```python
from build123d import *

# Parameters (mm, degrees)
F1_DEPTH      = 25.4
F1_DEPTH_BACK = 25.4
F3_D          = 5.1054


with BuildPart() as f1:
    # F0 (on Front) → F1 (new body, two sides)
    with BuildSketch(Plane.XZ) as f1_sk:
        Polygon((733.425, 292.1), (-733.425, 292.1), (-733.425, -292.1), (-682.625, -292.1), (-682.625, 241.3), (682.625, 241.3), (682.625, -292.1), (733.425, -292.1), align=None)
    extrude(amount=F1_DEPTH)
    extrude(f1_sk.sketch, amount=-F1_DEPTH_BACK)

    # F3 (through all)
    with Locations(Plane.XZ.offset(25.4)):
        with Locations((-708.025, -50.8), (708.025, -50.8), (708.025, 69.85), (-708.025, 69.85)):
            Hole(F3_D / 2)


solid = f1.part
```
Can you work these out from the model? Positions are in its coordinate system, mm. A direction names the side the tool comes from. Coordinates: 2 decimals unless noted, no trailing zeros. Order: outer loops, then holes, each group sorted by start corner. A loop starts at its lowest first (then second) coordinate and runs counter-clockwise, first axis right, second up.
1. Thinking about a two-plate mould opening in X: for faces 3 (the face through (-10, 0, 241.3)), 4 (the face through (-708, 0, -292.1)), 5 (the face through (-733.425, 0, 4)), 6 (the face through (733.425, 0, -4)), which applies, +X half, -X half, draft (parallel to the pull), parting line (faces both ways), or undercut?
2. If we section it at A-A (z = -70.5): Please give me the cut outline in (x, y) (3 decimals), then the cut area to 3 significant figures.
3. If we section it at C-C (x = 276): Please give me the cut outline in (y, z), then the cut area to 3 significant figures.
4. I need wall thicknesses on line 1 (X direction, y = 0, z = 69) (3 decimals); line 2 (X direction, y = 18, z = 122) (3 decimals); line 3 (Z direction, x = -478, y = 13.5). Which ranges of each line are inside material? Lowest first, please.
5. If we section it at B-B (y = -4): Please give me the cut outline in (x, z) (3 decimals).
6. For faces 1 (the face through (-682.625, 0, -29)), 2 (the face through (708, 0, -292.1)), which set-ups out of +Z, -Z, +X, -X, +Y, -Y let a thin tool reach every point of the face, with its end or its side?
7. I'm going to push flat-ended pins straight in: pin 1 (15 mm diameter, centred on x = -262, y = -9.5, fed in from -Z); pin 2 (4 mm diameter, centred on x = 708.025, z = -50.8, fed in from +Y); pin 3 (6.5 mm diameter, centred on x = -708.025, z = 69.85, fed in from +Y). Where does each tip first touch, or does it pass through?
Entries:
1. face 3: undercut
1. face 4: draft
1. face 5: -X half
1. face 6: +X half
2. outline: (-733.425, -25.4) - (-682.625, -25.4) - (-682.625, 25.4) - (-733.425, 25.4) - close; (682.625, -25.4) - (733.425, -25.4) - (733.425, 25.4) - (682.625, 25.4) - close
2. area: 5,160 mm2
3. outline: (-25.4, 241.3) - (25.4, 241.3) - (25.4, 292.1) - (-25.4, 292.1) - close
3. area: 2,580 mm2
4. line 1: x = -733.425 to -710.432, -705.618 to -682.625, 682.625 to 705.618, 710.432 to 733.425
4. line 2: x = -733.425 to -682.625, 682.625 to 733.425
4. line 3: z = 241.3 to 292.1
5. outline: (-733.425, -292.1) - (-682.625, -292.1) - (-682.625, 241.3) - (682.625, 241.3) - (682.625, -292.1) - (733.425, -292.1) - (733.425, 292.1) - (-733.425, 292.1) - close; hole circle Ø5.105 at (-708.025, -50.8); hole circle Ø5.105 at (-708.025, 69.85); hole circle Ø5.105 at (708.025, -50.8); hole circle Ø5.105 at (708.025, 69.85)
6. face 1: -Z, +Y, -Y
6. face 2: -Z, +X, -X, +Y, -Y
7. pin 1: stops at z = 241.3
7. pin 2: passes through
7. pin 3: stops at y = 25.4
